from build123d import *

# Parameters (mm, degrees)
SKETCH1_W           = 78
SKETCH1_H           = 125
BOSS_EXTRUDE1_DEPTH = 8
SKETCH2_R           = 7.5
SKETCH2_R_2         = 3
CUT_EXTRUDE1_DEPTH  = 4
SKETCH3_R           = 7.5
CUT_EXTRUDE2_DEPTH  = 148.39402973
SKETCH4_W           = 125
SKETCH4_H           = 20
SKETCH4_R           = 1.5
BOSS_EXTRUDE2_DEPTH = 3
SKETCH5_R           = 1.5
CUT_EXTRUDE3_DEPTH  = 149.690954668
SKETCH8_W           = 125
SKETCH8_H           = 28
BOSS_EXTRUDE3_DEPTH = 3
SKETCH9_R           = 1.5
CUT_EXTRUDE5_DEPTH  = 150.976664852
FILLET2_R           = 10


with BuildPart() as part:
    # Sketch1 → Boss-Extrude1 (new body)
    with BuildSketch(Plane(origin=(0, 0, 0), x_dir=(1, 0, 0), z_dir=(0, 1, 0))):
        with Locations((39, 62.5)):
            Rectangle(SKETCH1_W, SKETCH1_H)
    extrude(amount=BOSS_EXTRUDE1_DEPTH)

    # Sketch2 → Cut-Extrude1 (cut)
    with BuildSketch(Plane(origin=(0, 8, 0), x_dir=(-1, 0, 0), z_dir=(0, 1, 0))):
        with Locations(Location((-41.5, -90, 0), (0, 0, 90))):
            Circle(SKETCH2_R)
        with Locations(Location((-62.5, -90, 0), (0, 0, 90))):
            Circle(SKETCH2_R_2)
        with Locations(Location((-52, -71.813466521, 0), (0, 0, 90))):
            Circle(SKETCH2_R_2)
        with Locations(Location((-31, -71.813466521, 0), (0, 0, 90))):
            Circle(SKETCH2_R_2)
        with Locations(Location((-20.5, -90, 0), (0, 0, 90))):
            Circle(SKETCH2_R_2)
        with Locations(Location((-31, -108.186533479, 0), (0, 0, 90))):
            Circle(SKETCH2_R_2)
        with Locations(Location((-52, -108.186533479, 0), (0, 0, 90))):
            Circle(SKETCH2_R_2)
    extrude(amount=-CUT_EXTRUDE1_DEPTH, mode=Mode.SUBTRACT)

    # Sketch3 → Cut-Extrude2 (cut, through all)
    with BuildSketch(Plane(origin=(0, 4, 0), x_dir=(1, 0, 0), z_dir=(0, 1, 0))):
        with Locations(Location((41.5, 90, 0), (0, 0, 270))):
            Circle(SKETCH3_R)
    extrude(amount=-CUT_EXTRUDE2_DEPTH, mode=Mode.SUBTRACT)

    # Sketch4 → Boss-Extrude2 (add)
    with BuildSketch(Plane(origin=(78, 0, 0), x_dir=(0, 0, -1), z_dir=(1, 0, 0))):
        with Locations((62.5, 18)):
            Rectangle(SKETCH4_W, SKETCH4_H)
        with Locations((11.692170277, 22)):
            Circle(SKETCH4_R, mode=Mode.SUBTRACT)
        with Locations((36.692170277, 22)):
            Circle(SKETCH4_R, mode=Mode.SUBTRACT)
        with Locations((61.692170277, 22)):
            Circle(SKETCH4_R, mode=Mode.SUBTRACT)
        with Locations((86.692170277, 22)):
            Circle(SKETCH4_R, mode=Mode.SUBTRACT)
        with Locations((111.692170277, 22)):
            Circle(SKETCH4_R, mode=Mode.SUBTRACT)
    extrude(amount=-BOSS_EXTRUDE2_DEPTH)

    # Sketch5 → Cut-Extrude3 (cut, through all)
    with BuildSketch(Plane(origin=(0, 8, 0), x_dir=(-1, 0, 0), z_dir=(0, 1, 0))):
        with Locations(Location((-62.5, -90, 0), (0, 0, 90))):
            Circle(SKETCH5_R)
        with Locations(Location((-52, -71.813466521, 0), (0, 0, 90))):
            Circle(SKETCH5_R)
        with Locations(Location((-31, -71.813466521, 0), (0, 0, 90))):
            Circle(SKETCH5_R)
        with Locations(Location((-20.5, -90, 0), (0, 0, 90))):
            Circle(SKETCH5_R)
        with Locations(Location((-31, -108.186533479, 0), (0, 0, 90))):
            Circle(SKETCH5_R)
        with Locations(Location((-52, -108.186533479, 0), (0, 0, 90))):
            Circle(SKETCH5_R)
    extrude(amount=-CUT_EXTRUDE3_DEPTH, mode=Mode.SUBTRACT)

    # Sketch8 → Boss-Extrude3 (add)
    with BuildSketch(Plane.ZY):
        with Locations((-62.5, 14)):
            Rectangle(SKETCH8_W, SKETCH8_H)
    extrude(amount=BOSS_EXTRUDE3_DEPTH)

    # Sketch9 → Cut-Extrude5 (cut, through all)
    with BuildSketch(Plane(origin=(0, 0, 0), x_dir=(0, 0, -1), z_dir=(1, 0, 0))):
        with Locations((11.692170277, 22)):
            Circle(SKETCH9_R)
        with Locations((36.692170277, 22)):
            Circle(SKETCH9_R)
        with Locations((61.692170277, 22)):
            Circle(SKETCH9_R)
        with Locations((86.692170277, 22)):
            Circle(SKETCH9_R)
        with Locations((111.692170277, 22)):
            Circle(SKETCH9_R)
    extrude(amount=-CUT_EXTRUDE5_DEPTH, mode=Mode.SUBTRACT)

    # Fillet2
    fillet2_edges = [part.edges().sort_by_distance(p)[0] for p in [
        (-3, 14, -125),
        (78, 14, -125),
        (78, 14, 0),
        (-3, 14, 0),
    ]]
    fillet(fillet2_edges, radius=FILLET2_R)


solid = part.part
Design review of the part built by this model. Coordinates are the model's own, in mm. A direction names the side the tool comes from. Give positions to 0.01 mm unless a question says otherwise; leave off trailing zeros. Loops run counter-clockwise (first coordinate to the right, second up) from the corner with the lowest first, then second, coordinate; pieces in that order, holes last. Notation, with made-up numbers: M 48,10 L 69,10 A16 cw 69,36 Z; hole C 61,-35.75 d6. An arc over 180 degrees is marked long. Answer as a JSON object with one key per item and string values.
Item 1: We need section C-C (z = -90). State the section outline as (x, y) points.
Output values:
{"outline": "M -3,0 L 19,0 L 19,4 L 17.5,4 L 17.5,8 L 0,8 L 0,28 L -3,28 Z; M 22,0 L 34,0 L 34,8 L 23.5,8 L 23.5,4 L 22,4 Z; M 49,0 L 61,0 L 61,4 L 59.5,4 L 59.5,8 L 49,8 Z; M 64,0 L 78,0 L 78,28 L 75,28 L 75,8 L 65.5,8 L 65.5,4 L 64,4 Z"}
Item 2: Mouldability with a two-part tool opening along Y and no side actions: class faces 1 (the face through (-1, 28, -63)), 2 (the face through (38, 0, -63)), 3 (the face through (76, 11, -4)), 4 (the face through (76.521, 23.014, -60.587)) as pulls with the +Y half, pulls with the -Y half, needs draft (parallel to the pull), parting line crosses it, or undercut.
Output values:
{"face 1": "pulls with the +Y half", "face 2": "pulls with the -Y half", "face 3": "needs draft", "face 4": "undercut"}
Item 3: Machinability: for faces 5 (the face through (75, 18, -62)), 6 (the face through (31.066, 2.028, -109.685)), 7 (the face through (20.6, 6, -93)), which of the approach directions +Z, -Z, +X, -X, +Y, -Y give a long, thin tool a straight path to every point of the face, cutting with its end or side? Answer none if there is none.
Output values:
{"face 5": "+Z, -Z, +Y", "face 6": "+Y, -Y", "face 7": "+Y"}
Item 4: We need section A-A (x = 41.5). State the section outline as (y, z) points.
Output values:
{"outline": "M 0,-125 L 8,-125 L 8,-97.5 L 0,-97.5 Z; M 0,-82.5 L 8,-82.5 L 8,0 L 0,0 Z"}
Item 5: Wall thickness on line 1 along X through (y, z) = (6.4, -90); line 2 along X through (y, z) = (15, -54.5); line 3 along Y through (x, z) = (43.5, -105): over which ranges is each line inside the solid? List them lowest first.
Output values:
{"line 1": "x = -3 to 17.5, 23.5 to 34, 49 to 59.5, 65.5 to 78", "line 2": "x = -3 to 0, 75 to 78", "line 3": "y = 0 to 8"}
Item 6: We need section B-B (y = 5.5). State the section outline as (x, z) points.
Output values:
{"outline": "M -3,-115 A10 ccw 7,-125 L 68,-125 A10 ccw 78,-115 L 78,-10 A10 ccw 68,0 L 7,0 A10 ccw -3,-10 Z; hole C 20.5,-90 d6; hole C 31,-108.19 d6; hole C 31,-71.81 d6; hole C 41.5,-90 d15; hole C 52,-108.19 d6; hole C 52,-71.81 d6; hole C 62.5,-90 d6"}
Item 7: For P1, Ø2.5, axis at x = 20.5, z = -90, coming from the -Y side; P2, Ø5, axis at x = 9, z = -77.5, coming from the +Y side; P3, Ø3, axis at x = 52, z = -107, coming from the +Y side, all flat-tipped, find the tip position at first contact; note any pin that passes through.
Output values:
{"P1": "passes through", "P2": "stops at y = 8", "P3": "stops at y = 4"}
Item 8: We need section D-D (x = 52). State the section outline as (y, z) points.
Output values:
{"outline": "M 0,-125 L 8,-125 L 8,-111.19 L 4,-111.19 L 4,-109.69 L 0,-109.69 Z; M 0,-106.69 L 4,-106.69 L 4,-105.19 L 8,-105.19 L 8,-74.81 L 4,-74.81 L 4,-73.31 L 0,-73.31 Z; M 0,-70.31 L 4,-70.31 L 4,-68.81 L 8,-68.81 L 8,0 L 0,0 Z"}
